Could you check a few things on this drawing? It's one solid part, dimensions in mm from its lowest x, y, z. Round coordinates to 2 decimals unless told otherwise and drop trailing zeros. Order: outer loops, then holes, each group sorted by start corner. A loop starts at its lowest first (then second) coordinate and runs counter-clockwise, first axis right, second up. Notation, with made-up numbers: (31.25, 7) - (86.25, 7) arc R9 cw to (86.25, 20) - close; hole circle Ø10 at (-15.75, 59). An arc over 180 degrees is marked (long way). Use one line per item in the form item = value.
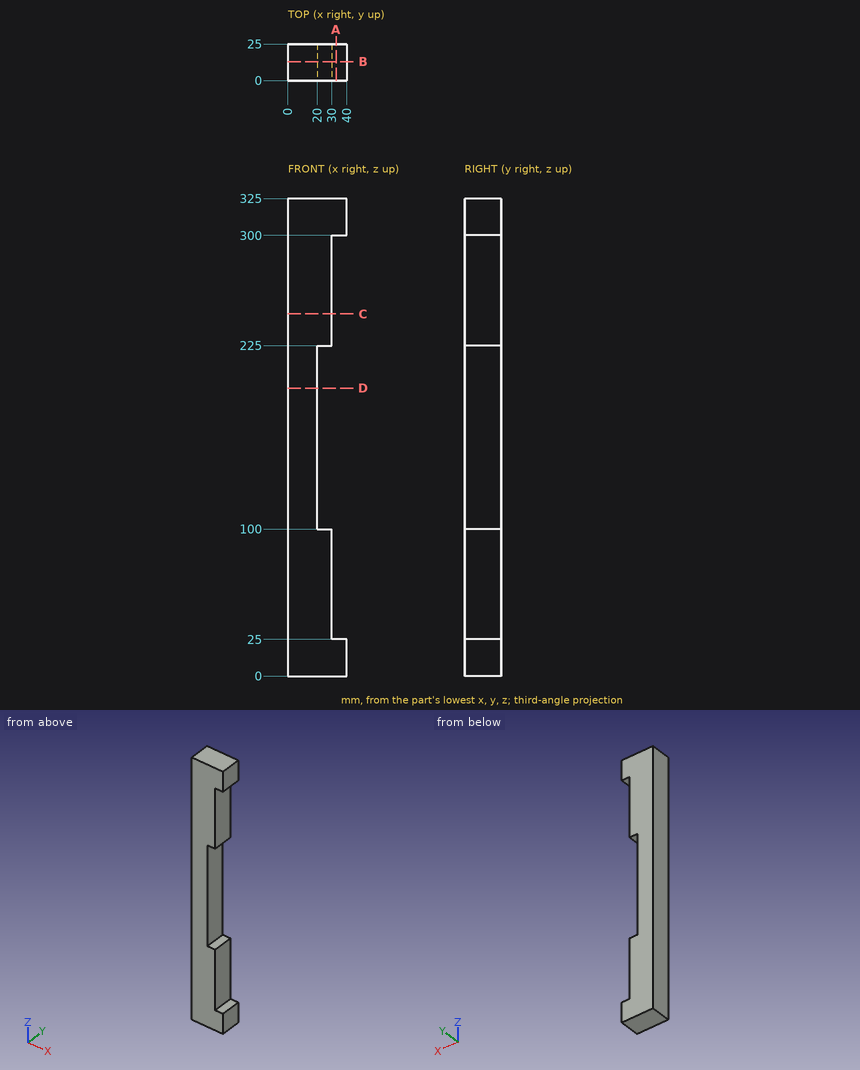
Item 1: Imagine slicing it at D-D on z = 196. Please give me the cut outline in (x, y).
Found:
outline = (0, 0) - (20, 0) - (20, 25) - (0, 25) - close
Item 2: Imagine slicing it at C-C on z = 246.5. Please give me the cut outline in (x, y).
Found:
outline = (0, 0) - (30, 0) - (30, 25) - (0, 25) - close
Item 3: Imagine slicing it at A-A on x = 33. Please give me the cut outline in (y, z), plus the area to 3 significant figures.
Found:
outline = (0, 0) - (25, 0) - (25, 25) - (0, 25) - close; (0, 300) - (25, 300) - (25, 325) - (0, 325) - close
area = 1,250 mm2
Item 4: Imagine slicing it at B-B on y = 13. Please give me the cut outline in (x, z).
Found:
outline = (0, 0) - (40, 0) - (40, 25) - (30, 25) - (30, 100) - (20, 100) - (20, 225) - (30, 225) - (30, 300) - (40, 300) - (40, 325) - (0, 325) - close
Item 5: Will these pins go through, and if not, where does the flat tip stop? P1, Ø3, axis at y = 14.5, z = 266.5, coming from the -X side; P2, Ø1.5, axis at y = 7, z = 78, coming from the +X side; P3, Ø12, axis at y = 11.5, z = 148.5, coming from the +X side.
Found:
P1 = 0
P2 = 30
P3 = 20
Item 6: I need wall thicknesses on L1, parallel to Z at x = 31, y = 12.25; L2, parallel to Z at x = 23, y = 21.75; L3, parallel to X at y = 19.5, z = 264. Which ranges of each line are inside material? Lowest first, please.
Found:
L1 = 0 to 25, 300 to 325
L2 = 0 to 100, 225 to 325
L3 = 0 to 30
